Could you check a few things on this model? Use its own coordinates, in mm. Face numbers are marked on the shaded views. Give positions to 0.01 mm unless a question says otherwise; leave off trailing zeros. Order: outer loops, then holes, each group sorted by start corner. A loop starts at its lowest first (then second) coordinate and runs counter-clockwise, first axis right, second up. Notation, with made-up numbers: (83, 75.5) -> (87, 75.5) arc R18 ccw to (87, 85.5) -> close; hole circle Ø8 at (41.5, 21). An arc over 180 degrees is marked (long way). Write each question's results on one line, items separated by ' | '.
Autodesk Inventor part; units mm, degrees
ref_plane "YZ Plane" through (0, 0, 0) normal (1, 0, 0) x (0, 1, 0)
ref_plane "XZ Plane" through (0, 0, 0) normal (0, 1, 0) x (-1, 0, 0)
ref_plane "XY Plane" through (0, 0, 0) normal (0, 0, 1) x (1, 0, 0)
sketch "Esboço1" plane through (0, 0, 0) normal (0, 1, 0) x (-1, 0, 0)
  arc A0 (-410, 0) -> (-289.9138, -289.9138) centre (0, 0) ccw
  arc A1 (-460, 0) -> (-325.2691, -325.2691) centre (0, 0) ccw
  circle A2 centre (0, 0) radius 460
  circle A3 centre (0, 0) radius 410
  line L0 (0, 0) -> (576.9105, 0)
  line L1 (0, 0) -> (-1224.3013, 0) construction
  line L2 (-410, 0) -> (-460, 0)
  point P0 (-460, 0)
  point P1 (-325.2691, -325.2691)
  point P2 (-289.9138, -289.9138)
  point P3 (-325.2691, -325.2691)
  point P4 (460, 0)
  point P5 (410, 0)
  point P6 (-289.9138, -289.9138)
  dimension "d27" = 820
  dimension "d28" = 920
  dimension "d87" = 180
extrude "Extrusão1" add sketch "Esboço1" along normal blind 6 contours A0 A3 L0 A2 A1 L2
sketch "Esboço6" plane through (0, 6, 0) normal (0, 1, 0) x (1, 0, 0)
  arc A0 (460, 0) -> (-460, 0) centre (0, 0) ccw
  circle A1 centre (0, 0) radius 460
  arc A2 (410, 0) -> (-410, 0) centre (0, 0) ccw
  circle A3 centre (0, 0) radius 410
  line L0 (0, 0) -> (743.005, 65.0045)
  line L1 (410, 0) -> (460, 0)
  line L2 (410, 0) -> (428, 0)
  line L3 (428, 0) -> (442, 0)
  line L4 (408.4398, 35.7339) -> (423.3827, 37.0412)
  line L5 (423.3827, 37.0412) -> (443.3066, 38.7843)
  line L6 (428, 0) -> (423.3827, 37.0412)
  line L7 (442, 0) -> (443.3066, 38.7843)
  point P0 (325.2691, 325.2691)
  point P1 (289.9138, 289.9138)
  dimension "d110" = -5
  dimension "d111" = 18
  dimension "d112" = 14
  dimension "d113" = 15
  dimension "d114" = 20
extrude "Extrusão6" cut sketch "Esboço6" against normal up to surface (6 mm away) contours L1 L6 L0 L7
sketch "Esboço8" plane through (0, 6, 0) normal (0, 1, 0) x (1, 0, 0)
  line L0 (0, 0) -> (-648.1086, -56.7022)
  line L1 (-460, 0) -> (-410, 0)
  arc A0 (460, 0) -> (-460, 0) centre (0, 0) ccw
  line L2 (-460, 0) -> (-442, 0)
  line L3 (-442, 0) -> (-428, 0)
  circle A1 centre (0, 0) radius 460
  circle A2 centre (0, 0) radius 410
  line L4 (-458.2496, -40.0916) -> (-443.3066, -38.7843)
  line L5 (-443.3066, -38.7843) -> (-423.3827, -37.0412)
  line L6 (-442, 0) -> (-443.3066, -38.7843)
  line L7 (-428, 0) -> (-423.3827, -37.0412)
  dimension "d137" = 5
  dimension "d138" = 18
  dimension "d139" = 14
  dimension "d140" = 15
  dimension "d141" = 20
extrude "Extrusão7" add sketch "Esboço8" against normal up to surface (6 mm away) contours L0 L6 L1 L7
equation "\"Raio_vergadura\" = Espessura"
equation "\"Largura_alívio_de_vergadura\" = Espessura"
equation "\"Profundidade_alívio_de_vergadura\" = 0.5 * Espessura"
equation "\"Tamanho_alívio_de_dobra\" = 4 * Espessura"
equation "\"Remanescente_mínimo\" = 2 * Espessura"
equation "\"Raiodetransição\" = Raio_vergadura"
equation "\"Tamanho_de_raio_de_Jacobi\" = Raio_vergadura"
equation "\"TamanhoFolga\" = Espessura"
properties part number "base"
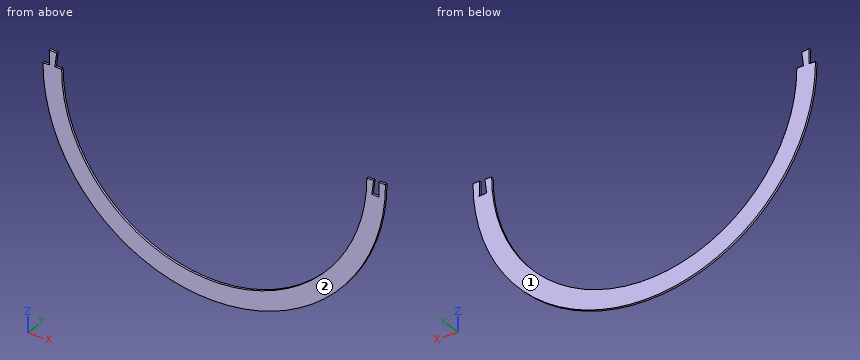
Q1. Thinking about a two-plate mould opening in Y: for the marked faces 1 and 2, which applies, +Y half, -Y half, draft (parallel to the pull), parting line (faces both ways), or undercut?
Here are the results:
face 1: +Y half | face 2: -Y half
Q2. I'm going to push flat-ended pins straight in: pin 1 Ø1.5 at (x, y) = (-132.5, 1) entering from -Z; pin 2 Ø3 at (x, y) = (-297, 3.5) entering from +Z; pin 3 Ø1.8 at (x, y) = (-419.5, 2) entering from +Z. Where does each tip first touch, or does it pass through?
Here are the results:
pin 1: stops at z = -440.73 | pin 2: stops at z = -281.07 | pin 3: stops at z = 0
Q3. Suppose I cut it at D-D on x = -93. Please give me the cut outline in (y, z), and give its area (3 significant figures).
Here are the results:
outline: (0, -450.5) -> (6, -450.5) -> (6, -399.31) -> (0, -399.31) -> close | area: 307 mm²
Q4. Suppose I cut it at B-B on y = 4.9. Please give me the cut outline in (x, z).
Here are the results:
outline: (-460, 0) arc R460 ccw to (325.27, -325.27) arc R460 ccw to (460, 0) -> (442, 0) -> (443.31, -38.78) -> (423.38, -37.04) -> (428, 0) -> (410, 0) arc R410 cw to (289.91, -289.91) arc R410 cw to (-410, 0) -> (-428, 0) -> (-423.38, 37.04) -> (-443.31, 38.78) -> (-442, 0) -> close
Q5. I need wall thicknesses on line 1 along X through (y, z) = (3.45, -125.5); line 2 along X through (y, z) = (3.4, -363.5); line 3 along Z through (x, y) = (-217, 4.9). Which ranges of each line are inside material? Lowest first, please.
Here are the results:
line 1: x = -442.55 to -390.32, 390.32 to 442.55 | line 2: x = -281.9 to -189.65, 189.65 to 281.9 | line 3: z = -405.6 to -347.87
Q6. Suppose I cut it at A-A on z = -121. Please give me the cut outline in (x, y), and give its area (3 significant figures).
Here are the results:
outline: (-443.8, 0) -> (-391.74, 0) -> (-391.74, 6) -> (-443.8, 6) -> close; (391.74, 0) -> (443.8, 0) -> (443.8, 6) -> (391.74, 6) -> close | area: 625 mm²
Q7. Suppose I cut it at C-C on z = -207.5. Please give me the cut outline in (x, y).
Here are the results:
outline: (-410.54, 0) -> (-353.62, 0) -> (-353.62, 6) -> (-410.54, 6) -> close; (353.62, 0) -> (410.54, 0) -> (410.54, 6) -> (353.62, 6) -> close
